Geometry: final body of the model. Coordinates: model frame, mm. A direction names the side the tool comes from. Give positions to 0.01 mm unless a question says otherwise; leave off trailing zeros. Write each loop counter-clockwise with the first axis right and the second up, starting at its lowest first coordinate (ties: lowest second). Pieces come first, ordered by that corner, then holes. Notation, with made-up numbers: M -32,-34 L 3,-34 A24 ccw 3,-7 Z; hole C 8,8.5 d4. An arc over 180 degrees is marked long. Use a Markdown table: item, result. Add a question column.
1) Section A-A on x = 321.5. Return the cut outline in (y, z), then the cut area to 3 significant figures.
2) Draft query along Z for faces 1 (the flat face through (291, 0, -8)), 2 (the flat face through (291, -6, 0)), 3 (the flat face through (188, -8, 0)), 4 (the flat face through (291, 6, 0)). Return one class per face: +Z half, -Z half, draft (parallel to the pull), parting line (faces both ways), or undercut.
3) Section B-B on z = 0.5. Return the cut outline in (x, y).
4) Set-up query: faces 5 (the flat face through (381.62, 7, 0)), 6 (the flat face through (93, 0, -6)). Return all of +Z, -Z, +X, -X, +Y, -Y with unobstructed straight access to the full face (end or side cutting, diameter ignored); none if empty.
5) Line query: line 1 (Z direction, x = 143, y = 0.5); line 2 (Y direction, x = 200, z = 0.75). Output: solid intervals per line, ascending.
6) Section C-C on y = 3.25. Return the cut outline in (x, z), then the cut area to 3 significant figures.
7) Section D-D on x = 200. Return the cut outline in (y, z).
Autodesk Inventor part; units mm, degrees
ref_plane "Work Plane1" through (0, -8, 8) normal (0.866, 0.5, 0) x (-0.5, 0.866, 0)
ref_plane "YZ Plane" through (0, 0, 0) normal (1, 0, 0) x (0, 1, 0)
ref_plane "XZ Plane" through (0, 0, 0) normal (0, 1, 0) x (-1, 0, 0)
sketch "Sketch1" plane through (0, 0, 0) normal (1, 0, 0) x (0, 1, 0)
  line L0 (6, 8) -> (-6, 8)
  line L1 (-8, 6) -> (-8, -6)
  line L2 (-6, -8) -> (6, -8)
  line L3 (8, -6) -> (8, 6)
  line L4 (8, 8) -> (-8, -8) construction
  line L5 (-8, 8) -> (8, -8) construction
  line L6 (6, -6) -> (-6, -6)
  line L7 (-6, -6) -> (-6, 6)
  line L8 (-6, 6) -> (6, 6)
  line L9 (6, 6) -> (6, -6)
  arc A0 (8, 6) -> (6, 8) centre (6, 6) ccw
  arc A1 (6, -8) -> (8, -6) centre (6, -6) ccw
  arc A2 (-8, -6) -> (-6, -8) centre (-6, -6) ccw
  arc A3 (-6, 8) -> (-8, 6) centre (-6, 6) ccw
  point P0 (0, 0)
  dimension "d1" = 16
  dimension "d2" = 16
  dimension "d3" = 2
  dimension "d4" = 2
extrude "Extrusion1" add sketch "Sketch1" along normal blind 381.62
sketch "Sketch2" plane through (0, -6, 8) normal (0, 0, 1) x (1, 0, 0)
  line L0 (0, 12) -> (0, 0)
  point P0 (0, 6)
  point P1 (200, 6)
  point P2 (0, 6)
  dimension "d7" = 200
hole "Hole1" at (200, 0, 8) direction (0, 0, -1) diameter 14 end through all
sketch "Sketch3" plane through (0, -6, 8) normal (0, 0, 1) x (1, 0, 0)
  line L0 (0, -2) -> (-9.2376, 14)
  line L1 (0, -2) -> (18.4752, -2) construction
  line L2 (-9.2376, 14) -> (0, 14)
  point P0 (0, 6)
  dimension "d15" = 120
ref_plane "Work Plane1" through (0, -8, 8) normal (0.866, 0.5, 0) x (-0.5, 0.866, 0)
extrude "Extrusion2" add sketch "Sketch1" against normal up to surface surface through (0, -8, 8) normal (0.866, 0.5, 0)
properties part number "suspensionarms"
Found:
| question | item | result |
|---|---|---|
| 1 | outline | M -8,-6 A2 ccw -6,-8 L 6,-8 A2 ccw 8,-6 L 8,6 A2 ccw 6,8 L -6,8 A2 ccw -8,6 Z; hole M -6,-6 L 6,-6 L 6,6 L -6,6 Z |
| 1 | area | 109 mm² |
| 2 | face 1 | -Z half |
| 2 | face 2 | undercut |
| 2 | face 3 | draft |
| 2 | face 4 | undercut |
| 3 | outline | M -9.24,8 L -8.08,6 L 196.39,6 A7 cw 203.61,6 L 381.62,6 L 381.62,8 Z; M -1.15,-6 L 0,-8 L 381.62,-8 L 381.62,-6 L 203.61,-6 A7 cw 196.39,-6 Z |
| 4 | face 5 | +Z, -Z, +X, +Y, -Y |
| 4 | face 6 | +X, -X |
| 5 | line 1 | -8 to -6, 6 to 8 |
| 5 | line 2 | -8 to -7, 7 to 8 |
| 6 | outline | M -6.5,-8 L 193.8,-8 L 193.8,-6 L -6.5,-6 Z; M -6.5,6 L 193.8,6 L 193.8,8 L -6.5,8 Z; M 206.2,-8 L 381.62,-8 L 381.62,-6 L 206.2,-6 Z; M 206.2,6 L 381.62,6 L 381.62,8 L 206.2,8 Z |
| 6 | area | 1,500 mm² |
| 7 | outline | M -8,-6 A2 ccw -7,-7.73 L -7,7.73 A2 ccw -8,6 Z; M 7,-7.73 A2 ccw 8,-6 L 8,6 A2 ccw 7,7.73 Z |
